```python
from build123d import *

# Parameters (mm, degrees)
SCHIZZO2_R                   = 6
ESTRUSIONE_ESTRUSIONE1_DEPTH = 11.5
SCHIZZO3_R                   = 7
ESTRUSIONE_ESTRUSIONE2_DEPTH = 4
ESTRUSIONE_ESTRUSIONE3_DEPTH = 26
RACCORDO2_R                  = 1.5
SCHIZZO6_R                   = 6.5
TAGLIO_ESTRUSIONE2_DEPTH     = 61.149812967
SMUSSO2_SIZE                 = 0.5


with BuildPart() as part:
    # Schizzo2 → Estrusione-Estrusione1 (new body)
    with BuildSketch(Plane.XY):
        Circle(SCHIZZO2_R)
    estrusione_estrusione1 = extrude(amount=ESTRUSIONE_ESTRUSIONE1_DEPTH)

    # Schizzo3 → Estrusione-Estrusione2 (add)
    with BuildSketch(Plane.XY.offset(11.5)):
        Circle(SCHIZZO3_R)
    estrusione_estrusione2 = extrude(amount=ESTRUSIONE_ESTRUSIONE2_DEPTH)

    # Schizzo4 → Estrusione-Estrusione3 (add)
    with BuildSketch(Plane.XY.offset(15.5)):
        with BuildLine():
            Line((-9.367496998, 7.5), (9.367496998, 7.5))
            ThreePointArc((9.367496998, 7.5), (12, 0), (9.367496998, -7.5))
            Line((9.367496998, -7.5), (-9.367496998, -7.5))
            ThreePointArc((-9.367496998, -7.5), (-12, 0), (-9.367496998, 7.5))
        make_face()
    extrude(amount=ESTRUSIONE_ESTRUSIONE3_DEPTH)

    # Specchia1: Estrusione-Estrusione2 across plane
    add(estrusione_estrusione2.mirror(Plane.XY.offset(28.5)))

    # Specchia2: Estrusione-Estrusione1 across plane
    add(estrusione_estrusione1.mirror(Plane.XY.offset(28.5)))

    # Raccordo2
    # the kernel refuses this fillet: 1.5 mm, written as the material it adds along each edge
    with BuildSketch(Plane(origin=(0, 0, 45.5), x_dir=(1, 0, 0), z_dir=(0, -1, 0))) as raccordo2_piece_1:
        with BuildLine():
            CenterArc((7.5, 1.414213562), RACCORDO2_R, 180, 70.528779366)
            Line((6, 1.414213562), (5.97, 1.414213562))
            Line((5.97, 1.414213562), (5.97, 0))
            Line((5.97, 0), (6, -0.03))
            ThreePointArc((6, -0.03), (6.5, -0.03), (6.99, -0.028284271))
            Line((6.99, -0.028284271), (7, 0))
        make_face()
    revolve(axis=Axis((0, 0, 45.5), (0, 0, 1)))
    with BuildSketch(Plane(origin=(0, 0, 11.5), x_dir=(1, 0, 0), z_dir=(0, -1, 0))) as raccordo2_piece_2:
        with BuildLine():
            CenterArc((7.5, -1.414213562), RACCORDO2_R, 109.471220634, 70.528779366)
            Line((6, -1.414213562), (5.97, -1.414213562))
            Line((5.97, -1.414213562), (5.97, 0))
            Line((5.97, 0), (6, 0.03))
            ThreePointArc((6, 0.03), (6.5, 0.03), (6.99, 0.028284271))
            Line((6.99, 0.028284271), (7, 0))
        make_face()
    revolve(axis=Axis((0, 0, 11.5), (0, 0, 1)))

    # Schizzo6 → Taglio-Estrusione2 (cut, through all)
    with BuildSketch(Plane(origin=(0, 7.5, 0), x_dir=(1, 0, 0), z_dir=(0, 1, 0))):
        with Locations(Location((0, -28.5, 0), (0, 0, 270))):
            Circle(SCHIZZO6_R)
    extrude(amount=-TAGLIO_ESTRUSIONE2_DEPTH, mode=Mode.SUBTRACT)

    # Smusso2
    smusso2_edges = [part.edges().sort_by_distance(p)[0] for p in [
        (0, -7.5, 22),
        (0, 7.5, 22),
    ]]
    chamfer(smusso2_edges, length=SMUSSO2_SIZE)


solid = part.part
```
Here's how the part is built. I have some questions about the finished solid (model axes, mm). A direction names the side the tool comes from. Coordinates: 2 decimals unless noted, no trailing zeros. Loops run counter-clockwise (first coordinate to the right, second up) from the corner with the lowest first, then second, coordinate; pieces in that order, holes last. Notation, with made-up numbers: M 31,57.5 L 85,57.5 A5 ccw 85,66.5 Z; hole C 27,5.5 d11. An arc over 180 degrees is marked long. One line per item, written item: value.
1. Imagine slicing it at B-B (x = 0). List the corners of the cut face in (y, z) for me, and give its area (3 significant figures).
Geometry says:
outline: M -7.5,15.5 L -7,15.5 L -7,11.5 A1.5 cw -6,10.09 L -6,0 L 6,0 L 6,10.09 A1.5 cw 7,11.5 L 7,15.5 L 7.5,15.5 L 7.5,21.5 L 7,22 L -7,22 L -7.5,21.5 Z; M -7.5,35.5 L -7,35 L 7,35 L 7.5,35.5 L 7.5,41.5 L 7,41.5 L 7,45.5 A1.5 cw 6,46.91 L 6,57 L -6,57 L -6,46.91 A1.5 cw -7,45.5 L -7,41.5 L -7.5,41.5 Z
area: 584 mm2
2. Imagine slicing it at C-C (z = 28.5). List the corners of the cut face in (x, y) for me, and give its area (3 significant figures).
Geometry says:
outline: M -9.37,-7.5 L -7,-7.5 L -6.5,-7 L -6.5,7 L -7,7.5 L -9.37,7.5 A12 ccw Z; M 6.5,-7 L 7,-7.5 L 9.37,-7.5 A12 ccw 9.37,7.5 L 7,7.5 L 6.5,7 Z
area: 139 mm2
3. Thinking about a two-plate mould opening in Z: for faces 4 (the cylindrical face through (0, 0, 22)), 5 (the flat face through (-2, -7, 41.5)), 6 (the cylindrical face through (12, 0, 28)), which applies, +Z half, -Z half, draft (parallel to the pull), parting line (faces both ways), or undercut?
Geometry says:
face 4: undercut
face 5: +Z half
face 6: draft
4. Will these pins go through, and if not, where does the flat tip stop? pin 1 Ø4 at (x, y) = (-8, -5.5) entering from -Z; pin 2 Ø6 at (y, z) = (-4, 26) entering from +X; pin 3 Ø2 at (y, z) = (-2, 47.5) entering from -X; pin 4 Ø10.5 at (x, z) = (0, 28.5) entering from -Y.
Geometry says:
pin 1: stops at z = 15.5
pin 2: stops at x = 11.96
pin 3: stops at x = -5.92
pin 4: passes through
5. Imagine slicing it at A-A (y = 0). List the corners of the cut face in (x, z) for me.
Geometry says:
outline: M -12,15.5 L -7,15.5 L -7,11.5 A1.5 cw -6,10.09 L -6,0 L 6,0 L 6,10.09 A1.5 cw 7,11.5 L 7,15.5 L 12,15.5 L 12,41.5 L 7,41.5 L 7,45.5 A1.5 cw 6,46.91 L 6,57 L -6,57 L -6,46.91 A1.5 cw -7,45.5 L -7,41.5 L -12,41.5 Z; hole C 0,28.5 d13
6. Please list where these lines run through material, in increasing order: probe 1 along X at (y, z) = (0.5, 28.5); probe 2 along Z at (x, y) = (-7.25, 5.5); probe 3 along Z at (x, y) = (-4, 3).
Geometry says:
probe 1: x = -11.99 to -6.5, 6.5 to 11.99
probe 2: z = 15.5 to 41.5
probe 3: z = 0 to 23.38, 33.62 to 57
7. On a 3-axis mill with a long thin cutter (end or side, diameter ignored), from which of +Z, -Z, +X, -X, +Y, -Y can I reach the whole of each face in a straight line? I mean faces 1 (the cylindrical face through (6.466, -2.681, 43.528)), 2 (the flat face through (-2, -7, 15.5)), 3 (the cylindrical face through (-12, 0, 28)). Say none if no direction works.
Geometry says:
face 1: +Z
face 2: -Z
face 3: +Z, -Z, -X
8. Imagine slicing it at D-D (z = 37). List the corners of the cut face in (x, y) for me.
Geometry says:
outline: M -9.37,-7.5 L 9.37,-7.5 A12 ccw 9.37,7.5 L -9.37,7.5 A12 ccw Z
